from build123d import *

# Parameters (mm, degrees)
PAD_DEPTH       = 1.02
SKETCH001_W     = 1.27
SKETCH001_H     = 1.07
POCKET_DEPTH    = 1.27
SKETCH002_W     = 1.27
SKETCH002_H     = 1.07
POCKET001_DEPTH = 1.27


with BuildPart() as part:
    # Sketch → Pad (new body)
    with BuildSketch(Plane.XY.offset(0.28)):
        Polygon((0, 0.94), (0.94, 0), (54.84, 0), (55.78, 0.94), (55.78, 13.74), (54.84, 14.68), (0.94, 14.68), (0, 13.74), align=None)
    extrude(amount=PAD_DEPTH)

    # Sketch001 → Pocket (cut)
    with BuildSketch(Plane(origin=(0, 0, 0.28), x_dir=(1, 0, 0), z_dir=(0, -1, 0))):
        with Locations((5.025, 0.535)):
            Rectangle(SKETCH001_W, SKETCH001_H)
        with Locations((7.565, 0.535)):
            Rectangle(SKETCH001_W, SKETCH001_H)
        with Locations((10.105, 0.535)):
            Rectangle(SKETCH001_W, SKETCH001_H)
        with Locations((12.644979, 0.52763)):
            Rectangle(SKETCH001_W, SKETCH001_H)
        with Locations((15.184957, 0.535)):
            Rectangle(SKETCH001_W, SKETCH001_H)
        with Locations((17.724957, 0.535)):
            Rectangle(SKETCH001_W, SKETCH001_H)
        with Locations((20.264957, 0.535)):
            Rectangle(SKETCH001_W, SKETCH001_H)
        with Locations((22.804957, 0.535)):
            Rectangle(SKETCH001_W, SKETCH001_H)
        with Locations((25.344957, 0.535)):
            Rectangle(SKETCH001_W, SKETCH001_H)
        with Locations((27.884957, 0.535)):
            Rectangle(SKETCH001_W, SKETCH001_H)
        with Locations((30.424957, 0.535)):
            Rectangle(SKETCH001_W, SKETCH001_H)
        with Locations((32.964957, 0.535)):
            Rectangle(SKETCH001_W, SKETCH001_H)
        with Locations((35.504957, 0.535)):
            Rectangle(SKETCH001_W, SKETCH001_H)
        with Locations((38.044957, 0.535)):
            Rectangle(SKETCH001_W, SKETCH001_H)
        with Locations((40.584957, 0.535)):
            Rectangle(SKETCH001_W, SKETCH001_H)
        with Locations((43.124957, 0.535)):
            Rectangle(SKETCH001_W, SKETCH001_H)
        with Locations((45.664957, 0.535)):
            Rectangle(SKETCH001_W, SKETCH001_H)
        with Locations((48.204957, 0.535)):
            Rectangle(SKETCH001_W, SKETCH001_H)
        with Locations((50.744957, 0.535)):
            Rectangle(SKETCH001_W, SKETCH001_H)
    extrude(amount=-POCKET_DEPTH, mode=Mode.SUBTRACT)

    # Sketch002 → Pocket001 (cut)
    with BuildSketch(Plane(origin=(0, 14.68, 0.28), x_dir=(-1, 0, 0), z_dir=(0, 1, 0))):
        with Locations((-45.665, 0.535)):
            Rectangle(SKETCH002_W, SKETCH002_H)
        with Locations((-43.125, 0.535)):
            Rectangle(SKETCH002_W, SKETCH002_H)
        with Locations((-40.585, 0.535)):
            Rectangle(SKETCH002_W, SKETCH002_H)
        with Locations((-40.585, 0.535)):
            Rectangle(SKETCH002_W, SKETCH002_H)
        with Locations((-40.585, 0.535)):
            Rectangle(SKETCH002_W, SKETCH002_H)
        with Locations((-38.045, 0.535)):
            Rectangle(SKETCH002_W, SKETCH002_H)
        with Locations((-35.505, 0.535)):
            Rectangle(SKETCH002_W, SKETCH002_H)
        with Locations((-32.965, 0.535)):
            Rectangle(SKETCH002_W, SKETCH002_H)
        with Locations((-30.425, 0.535)):
            Rectangle(SKETCH002_W, SKETCH002_H)
        with Locations((-27.885, 0.535)):
            Rectangle(SKETCH002_W, SKETCH002_H)
        with Locations((-25.345, 0.535)):
            Rectangle(SKETCH002_W, SKETCH002_H)
        with Locations((-22.805, 0.535)):
            Rectangle(SKETCH002_W, SKETCH002_H)
        with Locations((-20.265, 0.535)):
            Rectangle(SKETCH002_W, SKETCH002_H)
        with Locations((-17.725, 0.535)):
            Rectangle(SKETCH002_W, SKETCH002_H)
        with Locations((-15.185, 0.535)):
            Rectangle(SKETCH002_W, SKETCH002_H)
        with Locations((-12.645, 0.535)):
            Rectangle(SKETCH002_W, SKETCH002_H)
        with Locations((-10.105, 0.535)):
            Rectangle(SKETCH002_W, SKETCH002_H)
        with Locations((-7.565, 0.535)):
            Rectangle(SKETCH002_W, SKETCH002_H)
        with Locations((-5.025, 0.535)):
            Rectangle(SKETCH002_W, SKETCH002_H)
        with Locations((-48.205, 0.535)):
            Rectangle(SKETCH002_W, SKETCH002_H)
        with Locations((-50.745, 0.535)):
            Rectangle(SKETCH002_W, SKETCH002_H)
    extrude(amount=-POCKET001_DEPTH, mode=Mode.SUBTRACT)


solid = part.part
For this review, take the finished solid that the model builds, in its own axes (mm). A direction names the side the tool comes from. Round coordinates to 2 decimals unless told otherwise and drop trailing zeros. Order: outer loops, then holes, each group sorted by start corner. A loop starts at its lowest first (then second) coordinate and runs counter-clockwise, first axis right, second up. Notation, with made-up numbers: (58.25, 46) -> (117.25, 46) arc R29 ccw to (117.25, 77) -> close; hole circle Ø2 at (62, -17). An arc over 180 degrees is marked (long way). Write item = value, one per line. Start each with the question number.
1) Take a section at A-A on x = 38. State the section outline as (y, z) points, plus the area to 3 significant figures.
2) Tool access review of faces 1 (the face through (48, 1.27, 1)), 2 (the face through (41, 13.41, 1)), 3 (the face through (0.46, 0.48, 0.78)): name each direction out of +Z, -Z, +X, -X, +Y, -Y from which nothing blocks a thin tool from reaching the whole face with its end or side.
3) To check wall thickness, follow line 1 (Y direction, x = 38, z = 0.95). State the ranges of the line that lie inside material, in increasing order. Write a range as from..to.
4) Insertion check: pin 1 (0.5 mm diameter, centred on x = 20.5, z = 0.5, fed in from +Y); pin 2 (0.5 mm diameter, centred on x = 20.5, z = 1, fed in from -Y). Each pin has a flat end and moves straight along its axis. Give the tip position at first contact, or say it passes through.
5) The part is to be moulded in two halves that separate along X. For faces 4 (the face through (34, 0, 1)), 5 (the face through (35.5, 1.27, 0.8)), 6 (the face through (0.48, 14.22, 0.78)), say which applies: +X half, -X half, draft (parallel to the pull), parting line (faces both ways), or undercut.
Verdict:
q1.outline = (1.27, 0.28) -> (13.41, 0.28) -> (13.41, 1.3) -> (1.27, 1.3) -> close
q1.area = 12.4 mm2
q2.face_1 = +Z, -Z, -Y
q2.face_2 = +Z, -Z, +Y
q2.face_3 = +Z, -Z, -X, -Y
q3.line_1 = 1.27..13.41
q4.pin_1 = 13.41
q4.pin_2 = 1.27
q5.face_4 = draft
q5.face_5 = undercut
q5.face_6 = -X half
